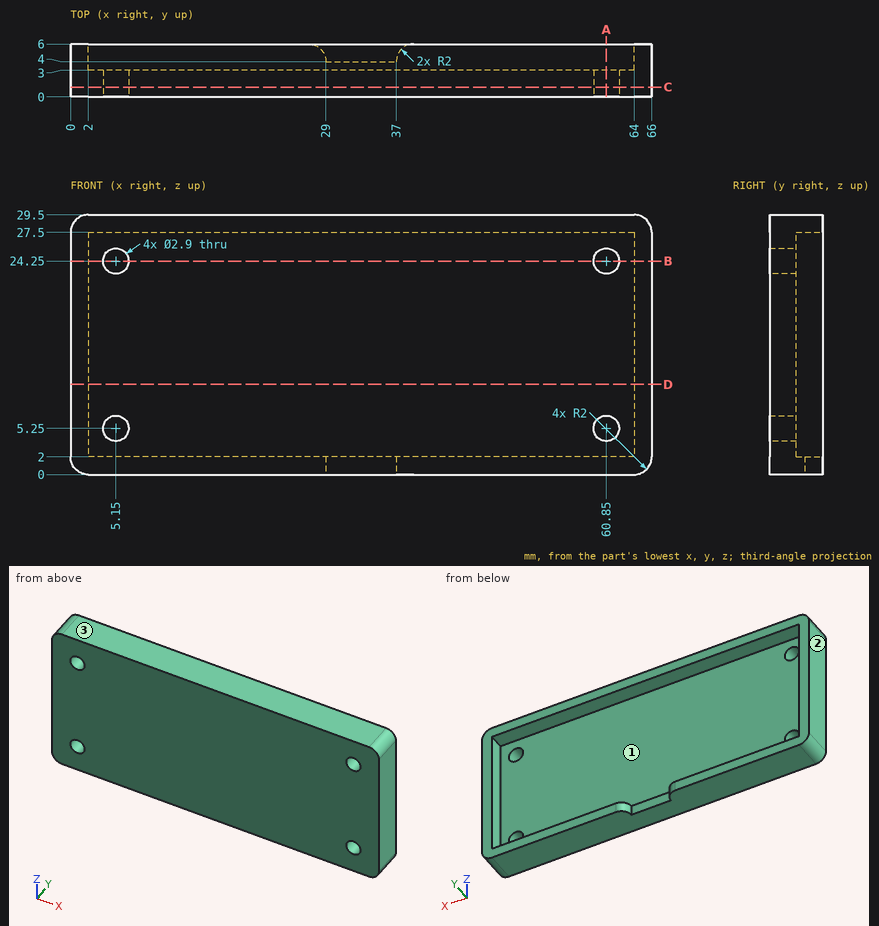
Geometry: see drawing. Coordinates: mm, zero at the bounding-box minimum. Give positions to 0.01 mm unless a question says otherwise; leave off trailing zeros. Loops run counter-clockwise (first coordinate to the right, second up) from the corner with the lowest first, then second, coordinate; pieces in that order, holes last. Notation, with made-up numbers: (48, 0) - (78, 0) arc R22 ccw to (78, 15) - close; hole circle Ø5 at (31.5, 85.5). An arc over 180 degrees is marked (long way). Use CSV: the item, a comma, the result in double quotes. Start each with the question number.
Item 1: Section D-D on z = 10.25. Return loops of the section in (x, y), then the cut area to 3 significant figures.
Item 2: Section B-B on z = 24.25. Return loops of the section in (x, y).
Item 3: Contact query for flat-ended pins moving along their axis: P1, Ø4, axis at x = 5.15, z = 5.25, coming from the -Y side; P2, Ø7.5, axis at x = 46, z = 21, coming from the +Y side; P3, Ø2, axis at x = 31, z = 1, coming from the +Y side. Output: stop coordinate, or through.
Item 4: Section A-A on x = 60.85. Return loops of the section in (y, z), then the cut area to 3 significant figures.
Item 5: Line query: line 1 (X direction, y = 1.1, z = 24.25); line 2 (Z direction, x = 42, y = 3.45); line 3 (X direction, y = 3.8, z = 16.25). Output: solid intervals per line, ascending.
Item 6: Mould query, pull axis Z, two halves, no side actions, for the marked faces 1, 2 and 3. Classes: pulls with the +Z half, pulls with the -Z half, needs draft (parallel to the pull), parting line crosses it, or undercut.
Item 7: Section C-C on y = 1.1. Return loops of the section in (x, z), then the cut area to 3 significant figures.
Ans:
1,outline,"(0, 0) - (66, 0) - (66, 6) - (64, 6) - (64, 3) - (2, 3) - (2, 6) - (0, 6) - close"
1,area,"210 mm2"
2,outline,"(0, 0) - (3.7, 0) - (3.7, 3) - (2, 3) - (2, 6) - (0, 6) - close; (6.6, 0) - (59.4, 0) - (59.4, 3) - (6.6, 3) - close; (62.3, 0) - (66, 0) - (66, 6) - (64, 6) - (64, 3) - (62.3, 3) - close"
3,P1,"stops at y = 0"
3,P2,"stops at y = 3"
3,P3,"stops at y = 4"
4,outline,"(0, 0) - (6, 0) - (6, 2) - (3, 2) - (3, 3.8) - (0, 3.8) - close; (0, 6.7) - (3, 6.7) - (3, 22.8) - (0, 22.8) - close; (0, 25.7) - (3, 25.7) - (3, 27.5) - (6, 27.5) - (6, 29.5) - (0, 29.5) - close"
4,area,"83.1 mm2"
5,line 1,"x = 0 to 3.7, 6.6 to 59.4, 62.3 to 66"
5,line 2,"z = 0 to 2, 27.5 to 29.5"
5,line 3,"x = 0 to 2, 64 to 66"
6,face 1,"undercut"
6,face 2,"needs draft"
6,face 3,"pulls with the +Z half"
7,outline,"(0, 2) arc R2 ccw to (2, 0) - (64, 0) arc R2 ccw to (66, 2) - (66, 27.5) arc R2 ccw to (64, 29.5) - (2, 29.5) arc R2 ccw to (0, 27.5) - close; hole circle Ø2.9 at (5.15, 5.25); hole circle Ø2.9 at (5.15, 24.25); hole circle Ø2.9 at (60.85, 5.25); hole circle Ø2.9 at (60.85, 24.25)"
7,area,"1,920 mm2"
